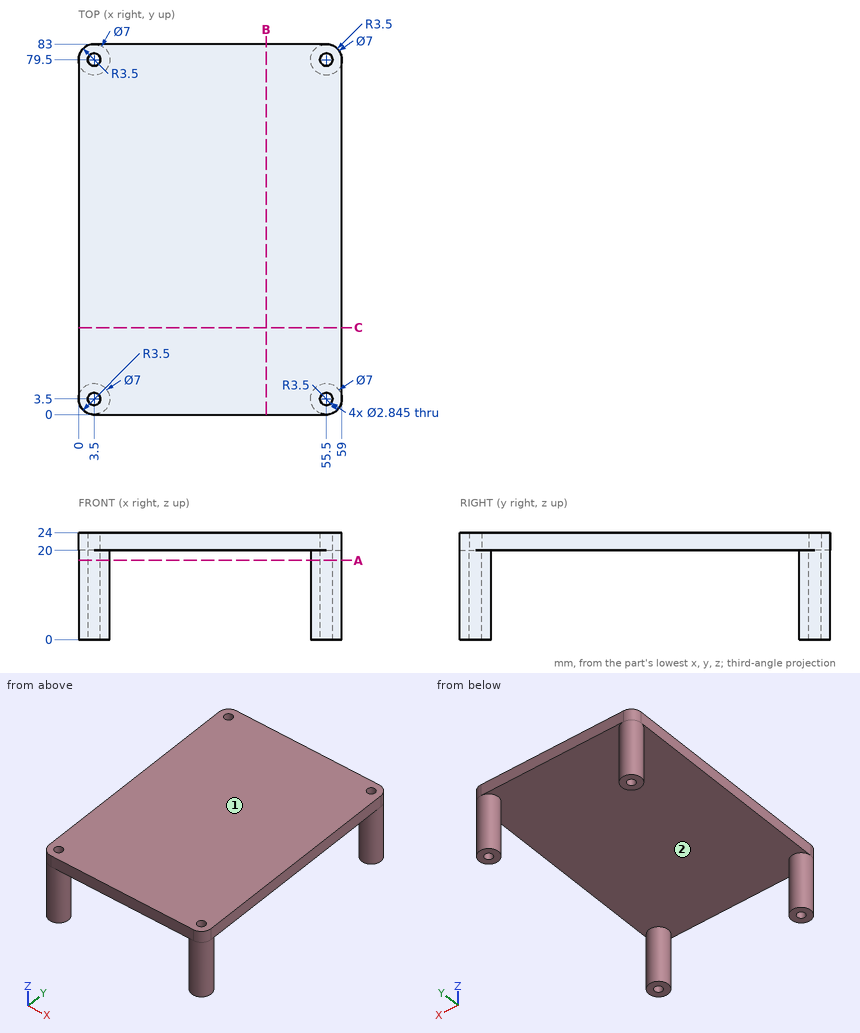
Here's the drawing with two shaded views (mm, measured from the low corner). I have some questions. Coordinates: 2 decimals unless noted, no trailing zeros. Loops run counter-clockwise (first coordinate to the right, second up) from the corner with the lowest first, then second, coordinate; pieces in that order, holes last. Notation, with made-up numbers: M 41,-9.75 L 79,-9.75 A21 ccw 79,-3.75 Z; hole C 33.5,55.5 d9. An arc over 180 degrees is marked long. Answer as CSV lines item,"result". Start each with the question number.
1. Thinking about a two-plate mould opening in Y: for the marked faces 1 and 2, which applies, +Y half, -Y half, draft (parallel to the pull), parting line (faces both ways), or undercut?
2. Suppose I cut it at C-C, the plane y = 19.5. List the corners of the cut face in (x, z) for me.
3. For pin 1 Ø3.5 at (x, y) = (55.5, 3.5) entering from -Z; pin 2 Ø2.5 at (x, y) = (3.5, 79.5) entering from -Z, each with a flat end and sliding along its axis, tell me the tip position at first contact or that it passes through.
4. If I drill on probe 1 along Y at (x, z) = (55.5, 4.5); probe 2 along Y at (x, z) = (55.5, 23.05); probe 3 along X at (y, z) = (79.5, 21.35), over which ranges is the centre line in solid material (lowest first)? Write a range as [from, to].
5. Suppose I cut it at A-A, the plane z = 17.75. List the corners of the cut face in (x, y) for me (1 decimal).
6. Suppose I cut it at B-B, the plane x = 42. List the corners of the cut face in (y, z) for me.
Output:
1,face 1,"draft"
1,face 2,"undercut"
2,outline,"M 0,20 L 59,20 L 59,24 L 0,24 Z"
3,pin 1,"stops at z = 0"
3,pin 2,"passes through"
4,probe 1,"y = [0, 2.08], [4.92, 7], [76, 78.08], [80.92, 83]"
4,probe 2,"y = [0, 2.08], [4.92, 78.08], [80.92, 83]"
4,probe 3,"x = [0, 2.08], [4.92, 54.08], [56.92, 59]"
5,outline,"C 3.5,3.5 d7; C 3.5,79.5 d7; C 55.5,3.5 d7; C 55.5,79.5 d7; hole C 3.5,3.5 d2.8; hole C 3.5,79.5 d2.8; hole C 55.5,3.5 d2.8; hole C 55.5,79.5 d2.8"
6,outline,"M 0,20 L 83,20 L 83,24 L 0,24 Z"
